from build123d import *

# Parameters (mm, degrees)
F0_R     = 38.1
F1_DEPTH = 101.6
F2_T     = -8.382
F3_R     = 5.08


# Not quite as in the source:
# - a fillet or chamfer that OpenCascade refuses, or shapes differently, is made with other operations: its cross-section is extruded or revolved along the edge and cut away or added


with BuildPart() as f1:
    # F0 (on Top) → F1 (new body)
    with BuildSketch(Plane.XY):
        Circle(F0_R)
    extrude(amount=F1_DEPTH)

    # F2
    f2_openings = [f1.faces().sort_by_distance(p)[0] for p in [
        (0, 0, 101.6),
    ]]
    offset(amount=F2_T, openings=f2_openings)

    # F3
    f3_edges = [f1.edges().sort_by_distance(p)[0] for p in [
        (-29.718, 0, 101.6),
    ]]
    fillet(f3_edges, radius=F3_R)

    # F4: fillet of radius 5.08 on 1 edges, made by hand

    # F4_s1 → F4_t2 (revolve, cut)
    with BuildSketch(Plane.XZ):
        with BuildLine():
            ThreePointArc((34.798, 101.6), (37.1936458882, 99.737357105), (38.1, 96.8413115252))
            Line((38.1, 96.8413115252), (38.1, 101.6))
            Line((38.1, 101.6), (34.798, 101.6))
        make_face()
    revolve(axis=Axis((0, 0, 101.6), (0, 0, 1)), mode=Mode.SUBTRACT)


solid = f1.part
The model under review builds one solid part; all positions refer to its coordinate system, in mm. Coordinates: 2 decimals unless noted, no trailing zeros. Loops run counter-clockwise (first coordinate to the right, second up) from the corner with the lowest first, then second, coordinate; pieces in that order, holes last. Notation, with made-up numbers: (40, 82.25) -> (85, 82.25) arc R17 cw to (85, 98.25) -> close; hole circle Ø1 at (69.25, 83). An arc over 180 degrees is marked (long way). Use a Markdown table: item, result. Add a question column.
1. Draft analysis for pull direction Y (two halves, no side actions). For faces 1 (the face through (-30.235, -23.183, 47.743)), 2 (the face through (-1, 1, 0)), 3 (the face through (0, 0, 8.382)), state which applies: pulls with the +Y half, pulls with the -Y half, needs draft (parallel to the pull), parting line crosses it, or undercut.
2. Clearance check with flat-ended pins moving along their axes: pin 1 Ø3 at (x, z) = (27.5, 14.5) entering from -Y; pin 2 Ø3 at (y, z) = (3, 88.5) entering from -X; pin 3 Ø6 at (x, y) = (-22, -4.5) entering from +Z. State where each tip first meets the part, or that it passes through.
3. Add section A-A on y = 0. Write out the cut boundary in (x, z), plus the area to 3 significant figures.
4. To check wall thickness, follow line 1 (Y direction, x = 0, z = 64); line 2 (Z direction, x = -1.5, y = 10.5); line 3 (Z direction, x = -33.5, y = 9.5). State the ranges of each line that lie inside material, in increasing order.
5. Add section C-C on z = 70. Write out the cut boundary in (x, y), plus the area to 3 significant figures.
Returned:
| question | item | result |
|---|---|---|
| 1 | face 1 | parting line crosses it |
| 1 | face 2 | needs draft |
| 1 | face 3 | undercut |
| 2 | pin 1 | stops at y = -27.85 |
| 2 | pin 2 | stops at x = -38.07 |
| 2 | pin 3 | stops at z = 8.38 |
| 3 | outline | (-38.1, 0) -> (38.1, 0) -> (38.1, 96.84) arc R5.08 ccw to (34.8, 101.6) arc R5.08 ccw to (29.72, 96.52) -> (29.72, 8.38) -> (-29.72, 8.38) -> (-29.72, 96.52) arc R5.08 ccw to (-34.8, 101.6) arc R5.08 ccw to (-38.1, 96.84) -> close |
| 3 | area | 2,180 mm² |
| 4 | line 1 | y = -38.1 to -29.72, 29.72 to 38.1 |
| 4 | line 2 | z = 0 to 8.38 |
| 4 | line 3 | z = 0 to 101.59 |
| 5 | outline | circle Ø76.2 at (0, 0); hole circle Ø59.44 at (0, 0) |
| 5 | area | 1,790 mm² |
